Geometry check sheet. Reference: the model listing, model coordinates, mm. Give positions to 0.01 mm unless a question says otherwise; leave off trailing zeros. Loops run counter-clockwise (first coordinate to the right, second up) from the corner with the lowest first, then second, coordinate; pieces in that order, holes last. Notation, with made-up numbers: (60.25, -7.5) -> (86.25, -7.5) arc R30 cw to (86.25, 19.5) -> close; hole circle Ø9 at (31, 54). An arc over 180 degrees is marked (long way). Write item = value, one per line. Start each with the question number.
```python
from build123d import *

# Parameters (mm, degrees)
SKETCH1_W      = 2.5
SKETCH1_H      = 25
REVOLVE1_ANGLE = 150
FILLET1_R      = 0.5


with BuildPart() as part:
    # Sketch1 → Revolve1 (revolve, symmetric)
    with BuildSketch(Plane(origin=(0, 0, 0), x_dir=(1, 0, 0), z_dir=(0, 1, 0))) as revolve1_sk:
        with Locations((-12.25, 0)):
            Rectangle(SKETCH1_W, SKETCH1_H)
    revolve(axis=Axis((0, 0, 0), (0, 0, -1)), revolution_arc=REVOLVE1_ANGLE / 2)
    revolve(revolve1_sk.sketch, axis=Axis((0, 0, 0), (0, 0, 1)), revolution_arc=REVOLVE1_ANGLE / 2)

    # Fillet1
    fillet1_edges = [part.edges().sort_by_distance(p)[0] for p in [
        (-2.847009496, 10.625184089, 0),
        (-3.170533303, 11.832591372, -12.5),
        (-3.170533303, -11.832591372, -12.5),
        (-3.494057109, -13.039998655, 0),
        (-3.170533303, -11.832591372, 12.5),
        (-3.494057109, 13.039998655, 0),
        (-2.847009496, -10.625184089, 0),
        (-13.5, 0, -12.5),
        (-11, 0, -12.5),
        (-11, 0, 12.5),
        (-13.5, 0, 12.5),
        (-3.170533303, 11.832591372, 12.5),
    ]]
    fillet(fillet1_edges, radius=FILLET1_R)


solid = part.part
```
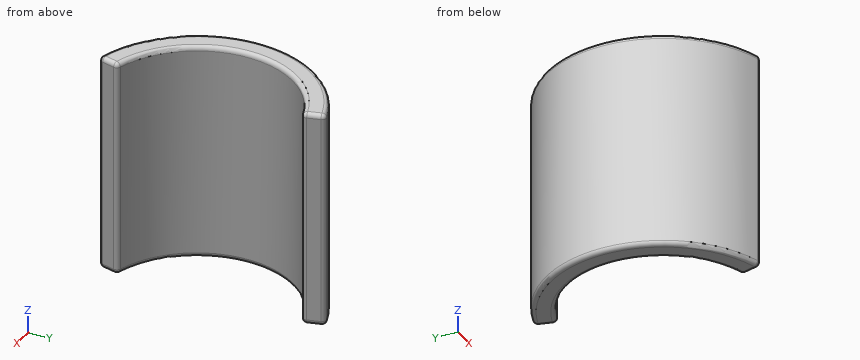
1) Thickness scan on line 1 (Y direction, x = -7.5, z = 11.5); line 2 (Y direction, x = -8.75, z = 8.5); line 3 (X direction, y = 0.25, z = 11). Record the ranges inside material, lowest first.
2) Depth check by flat-ended pin: pin 1 Ø1 at (y, z) = (1.5, 9.5) entering from +X; pin 2 Ø1.5 at (x, y) = (-10, -2) entering from +Z; pin 3 Ø2 at (x, z) = (-5, -8.5) entering from +Y; pin 4 Ø2 at (x, z) = (-12, -6.5) entering from +Y. Enter the tip coordinate at first touch or a pass-through.
3) Section check A-A (z = 6.25). Enter the section's corners in (x, y), plus the area to 3 significant figures.
Check result:
q1.line_1 = -11.22 to -8.05, 8.05 to 11.22
q1.line_2 = -10.28 to -6.67, 6.67 to 10.28
q1.line_3 = -13.5 to -11
q2.pin_1 = -10.82
q2.pin_2 = through
q2.pin_3 = 12.89
q2.pin_4 = 7.83
q3.outline = (-3.99, -12.9) arc R0.5 ccw to (-3.36, -12.55) -> (-2.97, -11.1) arc R0.5 ccw to (-3.31, -10.49) arc R11 cw to (-3.31, 10.49) arc R0.5 ccw to (-2.97, 11.1) -> (-3.36, 12.55) arc R0.5 ccw to (-3.99, 12.9) arc R13.5 ccw to start
q3.area = 80.0 mm2
